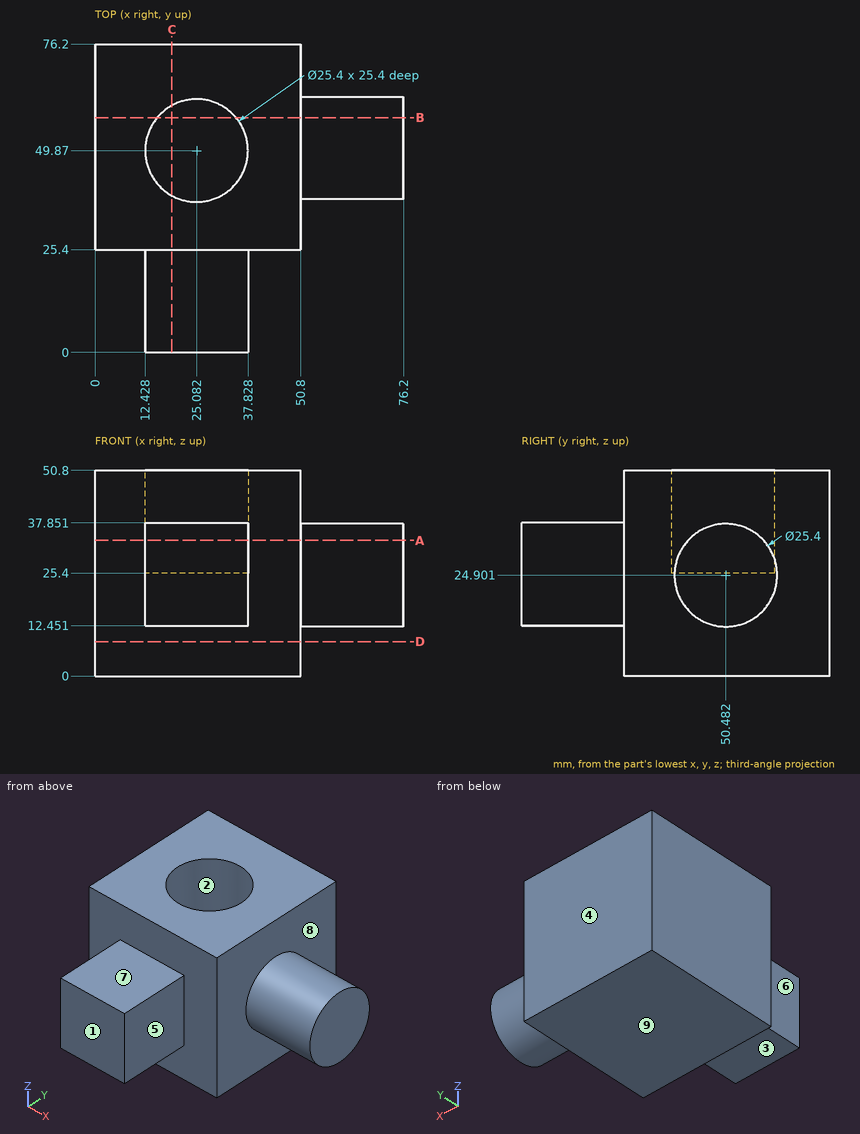
Here's the drawing with two shaded views (mm, measured from the low corner). I have some questions. A direction names the side the tool comes from. Give positions to 0.01 mm unless a question says otherwise; leave off trailing zeros. Loops run counter-clockwise (first coordinate to the right, second up) from the corner with the lowest first, then second, coordinate; pieces in that order, holes last. Notation, with made-up numbers: M 87.25,9.5 L 107.25,9.5 A25 ccw 107.25,31.5 Z; hole C 38.25,58.5 d3. An arc over 180 degrees is marked long. One line per item, written item: value.
(1) Suppose I cut it at D-D on z = 8.5. List the corners of the cut face in (x, y) for me, plus the area to 3 significant figures.
Returned:
outline: M 0,25.4 L 50.8,25.4 L 50.8,76.2 L 0,76.2 Z
area: 2,580 mm^2
(2) Suppose I cut it at B-B on y = 58. List the corners of the cut face in (x, z) for me (1 decimal).
Returned:
outline: M 0,0 L 50.8,0 L 50.8,14.7 L 76.2,14.7 L 76.2,35.1 L 50.8,35.1 L 50.8,50.8 L 34.8,50.8 L 34.8,25.4 L 15.3,25.4 L 15.3,50.8 L 0,50.8 Z
(3) Which directions (+Z, -Z, +X, -X, +Y, -Y) give clear straight access to the entire face, cutting with the end or side of a thin tool? Please do the marked faces 5, 6, 7, 8 and 9.
Returned:
face 5: +Z, -Z, +X, -Y
face 6: +Z, -Z, -X, -Y
face 7: +Z, +X, -X, -Y
face 8: +X
face 9: -Z, +X, -X, +Y, -Y
(4) Will these pins go through, and if not, where does the flat tip stop? pin 1 (4 mm diameter, centred on x = 62.5, z = 23.5, fed in from +Y); pin 2 (12.5 mm diameter, centred on x = 23, y = 53, fed in from +Z); pin 3 (7.5 mm diameter, centred on y = 18, z = 20, fed in from +X).
Returned:
pin 1: y = 63.18
pin 2: z = 25.4
pin 3: x = 37.83
(5) Suppose I cut it at C-C on x = 19. List the corners of the cut face in (y, z) for me.
Returned:
outline: M 0,12.45 L 25.4,12.45 L 25.4,0 L 76.2,0 L 76.2,50.8 L 61.02,50.8 L 61.02,25.4 L 38.72,25.4 L 38.72,50.8 L 25.4,50.8 L 25.4,37.85 L 0,37.85 Z
(6) I need wall thicknesses on line 1 (Z direction, x = 22, y = 47); line 2 (X direction, y = 8.5, z = 19); line 3 (Y direction, x = 42.5, z = 17). Which ranges of each line are inside material? Lowest first, please.
Returned:
line 1: 0 to 25.4
line 2: 12.43 to 37.83
line 3: 25.4 to 76.2
(7) We'd pull the mould along Y, two halves only. Please class the marked faces 1, 2, 3 and 4: released by +Y, released by -Y, zero draft, split by the parting line, or undercut.
Returned:
face 1: released by -Y
face 2: undercut
face 3: zero draft
face 4: released by +Y
(8) Suppose I cut it at A-A on z = 33.5. List the corners of the cut face in (x, y) for me, plus the area to 3 significant figures.
Returned:
outline: M 0,25.4 L 12.43,25.4 L 12.43,0 L 37.83,0 L 37.83,25.4 L 50.8,25.4 L 50.8,41.14 L 76.2,41.14 L 76.2,59.83 L 50.8,59.83 L 50.8,76.2 L 0,76.2 Z; hole C 25.08,49.87 d25.4
area: 3,190 mm^2
